Job drawing, mm, ordinate dimensions from the low corner. One solid piece. A direction names the side the tool comes from. Round coordinates to 2 decimals unless told otherwise and drop trailing zeros. Write each loop counter-clockwise with the first axis right and the second up, starting at its lowest first coordinate (ties: lowest second). Pieces come first, ordered by that corner, then holes.
1) Pull direction X, two halves, no side cores. Call the marked faces 1, 2, 3 and 4: +X half, -X half, draft (parallel to the pull), parting line (faces both ways), or undercut.
2) Saw through at C-C (z = 1.6). Write the cut outline in (x, y) (1 decimal).
3) Saw through at A-A (y = 4). Write the cut outline in (x, z).
4) Flat gauge pins, fed straight in: pin 1 (8 mm diameter, centred on x = 13, y = 21.5, fed in from +Z); pin 2 (3 mm diameter, centred on x = 23, z = 1.5, fed in from -Y). Where does each tip first touch, or does it go through?
5) Which spindle directions (+Z, -Z, +X, -X, +Y, -Y) get a long thin tool onto all of the face, cutting with end or side? Do the marked faces 5 and 6. Say none if no direction does.
6) Saw through at B-B (x = 9.75). Write the cut outline in (y, z), plus the area to 3 significant figures.
7) Wall check: probe 1 along Y at (x, z) = (23, 2.55); probe 2 along Y at (x, z) = (18.75, 3.8) (1 decimal); probe 3 along X at (y, z) = (14.5, 0.6) (1 decimal). Give the ranges that are in metal, low to high.
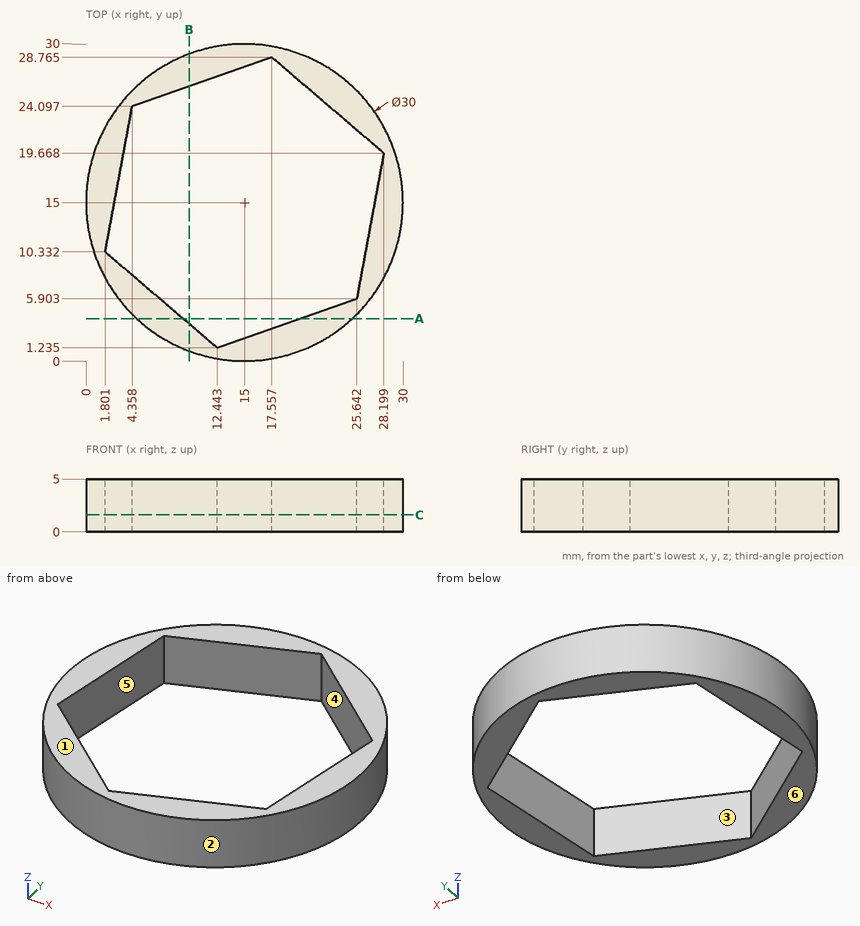
Evaluation:
1. face 1: draft
1. face 2: parting line
1. face 3: undercut
1. face 4: undercut
2. outline: circle Ø30 at (15, 15); hole (1.8, 10.3) - (12.4, 1.2) - (25.6, 5.9) - (28.2, 19.7) - (17.6, 28.8) - (4.4, 24.1) - close
3. outline: (4.8, 0) - (9.21, 0) - (9.21, 5) - (4.8, 5) - close; (20.26, 0) - (25.2, 0) - (25.2, 5) - (20.26, 5) - close
4. pin 1: passes through
4. pin 2: stops at y = 1.48
5. face 5: +Z, -Z
5. face 6: -Z, +X, -X, +Y, -Y
6. outline: (0.95, 0) - (3.54, 0) - (3.54, 5) - (0.95, 5) - close; (26, 0) - (29.05, 0) - (29.05, 5) - (26, 5) - close
6. area: 28.2 mm2
7. probe 1: y = 2.31 to 4.97, 24.11 to 27.69
7. probe 2: y = 0.5 to 3.5, 27.7 to 29.5
7. probe 3: x = 0 to 2.6, 27.2 to 30
